```python
from build123d import *

# Parameters (mm, degrees)
SKETCH1_R           = 9.525
BOSS_EXTRUDE1_DEPTH = 11.176
SKETCH3_R           = 8.509
BOSS_EXTRUDE3_DEPTH = 2.54
BOSS_EXTRUDE4_DEPTH = 8.89
SKETCH5_R           = 8.6614
BOSS_EXTRUDE5_DEPTH = 2.54
SKETCH6_R           = 9.525
BOSS_EXTRUDE6_DEPTH = 1.778
BOSS_EXTRUDE7_DEPTH = 14.478
SKETCH8_R           = 10.8712
BOSS_EXTRUDE8_DEPTH = 3.048
FILLET1_R           = 0.508
SKETCH9_R           = 6.4389
CUT_EXTRUDE1_DEPTH  = 48.580882343


with BuildPart() as part:
    # Sketch1 → Boss-Extrude1 (new body)
    with BuildSketch(Plane(origin=(0, 0, 0), x_dir=(1, 0, 0), z_dir=(0, 1, 0))):
        with Locations(Location((0, 0, 0), (0, 0, 270))):
            Circle(SKETCH1_R)
    extrude(amount=BOSS_EXTRUDE1_DEPTH)

    # Sketch3 → Boss-Extrude3 (add)
    with BuildSketch(Plane(origin=(0, 11.176, 0), x_dir=(1, 0, 0), z_dir=(0, 1, 0))):
        with Locations(Location((0, 0, 0), (0, 0, 270))):
            Circle(SKETCH3_R)
    extrude(amount=BOSS_EXTRUDE3_DEPTH)

    # Sketch4 → Boss-Extrude4 (add)
    with BuildSketch(Plane(origin=(0, 13.716, 0), x_dir=(1, 0, 0), z_dir=(0, 1, 0))):
        Polygon((12.831609733, 0), (6.415804866, 11.1125), (-6.415804866, 11.1125), (-12.831609733, 0), (-6.415804866, -11.1125), (6.415804866, -11.1125), align=None)
    extrude(amount=BOSS_EXTRUDE4_DEPTH)

    # Sketch5 → Boss-Extrude5 (add)
    with BuildSketch(Plane(origin=(0, 22.606, 0), x_dir=(1, 0, 0), z_dir=(0, 1, 0))):
        with Locations(Location((0, 0, 0), (0, 0, 270))):
            Circle(SKETCH5_R)
    extrude(amount=BOSS_EXTRUDE5_DEPTH)

    # Sketch6 → Boss-Extrude6 (add)
    with BuildSketch(Plane(origin=(0, 25.146, 0), x_dir=(1, 0, 0), z_dir=(0, 1, 0))):
        with Locations(Location((0, 0, 0), (0, 0, 270))):
            Circle(SKETCH6_R)
    extrude(amount=BOSS_EXTRUDE6_DEPTH)

    # Sketch7 → Boss-Extrude7 (add)
    with BuildSketch(Plane(origin=(0, 26.924, 0), x_dir=(1, 0, 0), z_dir=(0, 1, 0))):
        Polygon((-6.415804866, -11.1125), (6.415804866, -11.1125), (12.831609733, 0), (6.415804866, 11.1125), (-6.415804866, 11.1125), (-12.831609733, 0), align=None)
    extrude(amount=BOSS_EXTRUDE7_DEPTH)

    # Sketch8 → Boss-Extrude8 (add)
    with BuildSketch(Plane(origin=(0, 41.402, 0), x_dir=(1, 0, 0), z_dir=(0, 1, 0))):
        with Locations(Location((0, 0, 0), (0, 0, 90))):
            Circle(SKETCH8_R)
    extrude(amount=BOSS_EXTRUDE8_DEPTH)

    # Fillet1
    fillet1_edges = [part.edges().sort_by_distance(p)[0] for p in [
        (0, 44.45, 10.8712),
    ]]
    fillet(fillet1_edges, radius=FILLET1_R)

    # Sketch9 → Cut-Extrude1 (cut, through all)
    with BuildSketch(Plane(origin=(0, 44.45, 0), x_dir=(1, 0, 0), z_dir=(0, 1, 0))):
        with Locations(Location((0, 0, 0), (0, 0, 270))):
            Circle(SKETCH9_R)
    extrude(amount=-CUT_EXTRUDE1_DEPTH, mode=Mode.SUBTRACT)


solid = part.part
```
CAD build for the part. Positions are in the model's coordinates, mm. A direction names the side the tool comes from. Round coordinates to 2 decimals unless told otherwise and drop trailing zeros. Order: outer loops, then holes, each group sorted by start corner. A loop starts at its lowest first (then second) coordinate and runs counter-clockwise, first axis right, second up.
Q1. Which spindle directions (+Z, -Z, +X, -X, +Y, -Y) get a long thin tool onto all of the face, cutting with end or side? Do faces 4 (the flat face through (0, 34, -11.112)), 5 (the cylindrical face through (-5.796, 26.023, -7.559)). Say none if no direction does.
Q2. Drop flat-ended pins along their axis: pin 1 (2 mm diameter, centred on y = 29, z = 8, fed in from -X); pin 2 (1.5 mm diameter, centred on x = -10, y = 35, fed in from -Z); pin 3 (3 mm diameter, centred on y = 8.5, z = -5, fed in from -X). Give the stop position or say it passes through.
Q3. Slice it at D-D (y = 4.5). Write the cut outline in (x, z) (3 decimals).
Q4. Slice it at C-C (y = 23.5). Write the cut outline in (x, z).
Q5. Wall check: L1, parallel to X at y = 26, z = 0 (3 decimals); L2, parallel to X at y = 19.5, z = 0; L3, parallel to Y at x = 9.75, z = 1.25. Give the ranges that are in metal, low to high.
Q6. Two-plate mould, pull along Y, no slides. Class faces 1 (the flat face through (0, 44.45, -7)), 2 (the cylindrical face through (-7.684, 23.858, 3.997)), 3 (the flat face through (-9.6, 34.1, -5.6)): pulls with the +Y half, pulls with the -Y half, needs draft (parallel to the pull), parting line crosses it, or undercut.
Q7. Slice it at B-B (y = 40). Write the cut outline in (x, z).
Results below:
1. face 4: -Z, +X, -X, +Y, -Y
1. face 5: none
2. pin 1: stops at x = -8.79
2. pin 2: stops at z = -6.2
2. pin 3: stops at x = -8.86
3. outline: circle Ø19.05 at (0, 0); hole circle Ø12.878 at (0, 0)
4. outline: circle Ø17.32 at (0, 0); hole circle Ø12.88 at (0, 0)
5. L1: x = -9.525 to -6.439, 6.439 to 9.525
5. L2: x = -12.83 to -6.44, 6.44 to 12.83
5. L3: y = 13.72 to 22.61, 26.92 to 44.45
6. face 1: pulls with the +Y half
6. face 2: undercut
6. face 3: needs draft
7. outline: (-12.83, 0) - (-6.42, -11.11) - (6.42, -11.11) - (12.83, 0) - (6.42, 11.11) - (-6.42, 11.11) - close; hole circle Ø12.88 at (0, 0)
